For this review, take the finished solid that the model builds, in its own axes (mm). A direction names the side the tool comes from. Give positions to 0.01 mm unless a question says otherwise; leave off trailing zeros. Loops run counter-clockwise (first coordinate to the right, second up) from the corner with the lowest first, then second, coordinate; pieces in that order, holes last. Notation, with made-up numbers: (27.25, -25) - (33.25, -25) arc R19 cw to (33.25, -2) - close; hole circle Ø3 at (54, 82.25). An arc over 180 degrees is marked (long way). Answer in a Markdown table with one row per item.
```python
from build123d import *

# Parameters (mm, degrees)
SKETCH_1_R             = 1.6
SM_BASE_FLANGE_1_DEPTH = 0.9
OTHER_START            = -11
OTHER_1_DEPTH          = 22
OTHER_1_2_DEPTH        = 22


# Read off the part's stored shape, not the designer's step: 褶边1
# Sheet-metal steps are written as plain solids
with BuildPart() as part:
    # Sketch 1 → 基体-法兰1 (new body)
    with BuildSketch(Plane.XY):
        with BuildLine():
            Line((11, 0), (-11, 0))
            Line((-11, 0), (-11, 10))
            ThreePointArc((-11, 10), (0, 14.866068747), (11, 10))
            Line((11, 10), (11, 0))
        make_face()
        with Locations((-6.5, 6.5)):
            Circle(SKETCH_1_R, mode=Mode.SUBTRACT)
        with Locations(Location((6.5, 6.5, 0), (0, 0, 180))):
            Circle(SKETCH_1_R, mode=Mode.SUBTRACT)
    extrude(amount=-SM_BASE_FLANGE_1_DEPTH)

    # Other 1 outline → Other 1 (cut)
    with BuildSketch(Plane.YZ.offset(OTHER_START)):
        with BuildLine():
            ThreePointArc((2.4, -0.9), (1.360769515, -0.663330765), (0.5265006, 0))
            Line((0.5265006, 0), (0, 0))
            Line((0, 0), (0, -0.9))
            Line((0, -0.9), (2.4, -0.9))
        make_face()
    extrude(amount=OTHER_1_DEPTH, mode=Mode.SUBTRACT)

    # Other 1 2 outline → Other 1 2 (add)
    with BuildSketch(Plane.YZ.offset(OTHER_START)):
        with BuildLine():
            Line((2.4, 3), (2.4, 3.9))
            ThreePointArc((2.4, 3.9), (0.236669235, 2.539230485), (0.5265006, 0))
            Line((0.5265006, 0), (2.4, 0))
            ThreePointArc((2.4, 0), (0.9, 1.5), (2.4, 3))
        make_face()
    extrude(amount=OTHER_1_2_DEPTH)


solid = part.part
```
1. Mouldability with a two-part tool opening along X and no side actions: class faces 3 (the face through (-0.2, 0.9, 1.5)), 4 (the face through (5.76, 7.92, -0.44)), 5 (the face through (-11, 4.2, -0.3)), 6 (the face through (-6.85, 4.94, -0.44)) as released by +X, released by -X, zero draft, split by the parting line, or undercut.
Values:
| item | result |
|---|---|
| face 3 | zero draft |
| face 4 | undercut |
| face 5 | released by -X |
| face 6 | undercut |
2. Wall thickness on line 1 (Z direction, x = 2.5, y = 3); line 2 (Y direction, x = 6.5, z = -0.45); line 3 (Y direction, x = 6.5, z = -0.6): over which ranges is each line inside the solid? List them lowest first. Write a range as [from, to].
Values:
| item | result |
|---|---|
| line 1 | z = [-0.9, 0] |
| line 2 | y = [1, 4.9], [8.1, 13.37] |
| line 3 | y = [1.24, 4.9], [8.1, 13.37] |
3. We need section B-B, the plane x = 6.5. Give the boundary of the cut face in (y, z).
Values:
| item | result |
|---|---|
| outline | (2.4, -0.9) - (4.9, -0.9) - (4.9, 0) - (2.4, 0) arc R1.5 cw to (2.4, 3) - (2.4, 3.9) arc R2.4 ccw to start; (8.1, -0.9) - (13.37, -0.9) - (13.37, 0) - (8.1, 0) - close |
4. We need section D-D, the plane y = 9. Give the boundary of the cut face in (x, z), and give its area (3 significant figures).
Values:
| item | result |
|---|---|
| outline | (-11, -0.9) - (11, -0.9) - (11, 0) - (-11, 0) - close |
| area | 19.8 mm^2 |
5. Clearance check with flat-ended pins moving along their axes: pin 1 (3 mm diameter, centred on x = 3, y = 7.5, fed in from +Z); pin 2 (1.5 mm diameter, centred on x = 1.5, z = 2.5, fed in from -Y); pin 3 (1.9 mm diameter, centred on x = 6.5, y = 6.5, fed in from +Z) (3 decimals); pin 4 (1.5 mm diameter, centred on x = 7.5, z = 0.5, fed in from +Y). State where each tip first meets the part, or that it passes through.
Values:
| item | result |
|---|---|
| pin 1 | stops at z = 0 |
| pin 2 | stops at y = 0.01 |
| pin 3 | passes through |
| pin 4 | stops at y = 13.15 |
6. For faces 1 (the face through (-0.2, 2.4, 3.4)), 2 (the face through (-0.173, 14.865, -0.444)), list the 3-axis set-ups (+Z, -Z, +X, -X, +Y, -Y) from which the entire face can be reached by the end or side of a thin tool; tool diameter is ignored.
Values:
| item | result |
|---|---|
| face 1 | +Z, +X, -X, +Y |
| face 2 | +Z, -Z, +Y |
7. We need section A-A, the plane y = 6.5. Give the boundary of the cut face in (x, z), and give its area (3 significant figures).
Values:
| item | result |
|---|---|
| outline | (-11, -0.9) - (-8.1, -0.9) - (-8.1, 0) - (-11, 0) - close; (-4.9, -0.9) - (4.9, -0.9) - (4.9, 0) - (-4.9, 0) - close; (8.1, -0.9) - (11, -0.9) - (11, 0) - (8.1, 0) - close |
| area | 14.0 mm^2 |
8. We need section C-C, the plane x = 2.25. Give the boundary of the cut face in (y, z), and give its area (3 significant figures).
Values:
| item | result |
|---|---|
| outline | (2.4, -0.9) - (14.69, -0.9) - (14.69, 0) - (2.4, 0) arc R1.5 cw to (2.4, 3) - (2.4, 3.9) arc R2.4 ccw to start |
| area | 16.6 mm^2 |
